Work out the finished part from the listing and answer in its coordinate system (mm). Coordinates: 2 decimals unless noted, no trailing zeros. Loops run counter-clockwise (first coordinate to the right, second up) from the corner with the lowest first, then second, coordinate; pieces in that order, holes last. Notation, with made-up numbers: (35.5, 61.5) -> (72.5, 61.5) arc R27 cw to (72.5, 77.5) -> close; hole circle Ø3 at (25.5, -35.5). An arc over 180 degrees is marked (long way). One line per question, with ' | ' between items.
```python
from build123d import *

# Parameters (mm, degrees)
F1_DEPTH = 20.32


with BuildPart() as f1:
    # F0 (on Top) → F1 (new body)
    with BuildSketch(Plane.XY):
        with BuildLine():
            Line((190.5, -368.3), (215.9, -368.3))
            ThreePointArc((215.9, -368.3), (278.761793, -342.261793), (304.8, -279.4))
            Line((304.8, -279.4), (304.8, 279.4))
            ThreePointArc((304.8, 279.4), (278.761793, 342.261793), (215.9, 368.3))
            Line((215.9, 368.3), (-215.9, 368.3))
            ThreePointArc((-215.9, 368.3), (-278.761793, 342.261793), (-304.8, 279.4))
            Line((-304.8, 279.4), (-304.8, -279.4))
            ThreePointArc((-304.8, -279.4), (-278.761793, -342.261793), (-215.9, -368.3))
            Line((-215.9, -368.3), (-190.5, -368.3))
            Line((-190.5, -368.3), (190.5, -368.3))
        make_face()
    extrude(amount=F1_DEPTH)


solid = f1.part
```
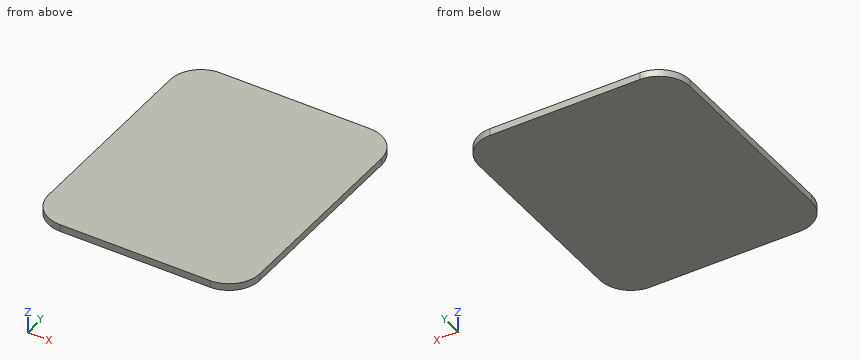
1) Find section A-A (z = 11.5). Write down the section's boundary in (x, y).
Check values:
outline: (-304.8, -279.4) arc R88.9 ccw to (-215.9, -368.3) -> (215.9, -368.3) arc R88.9 ccw to (304.8, -279.4) -> (304.8, 279.4) arc R88.9 ccw to (215.9, 368.3) -> (-215.9, 368.3) arc R88.9 ccw to (-304.8, 279.4) -> close
2) Find the intervals of material crossed by line 1 along X through (y, z) = (282, 1.25); line 2 along Y through (x, z) = (-263.5, 8.75); line 3 along X through (y, z) = (321, 2), in increasing order.
Check values:
line 1: x = -304.76 to 304.76 | line 2: y = -354.48 to 354.48 | line 3: x = -294.47 to 294.47
3) Find section B-B (x = 261.5). Write down the section's boundary in (y, z), plus the area to 3 significant figures.
Check values:
outline: (-355.71, 0) -> (355.71, 0) -> (355.71, 20.32) -> (-355.71, 20.32) -> close | area: 14,500 mm^2
